Here's the drawing with two shaded views (mm, measured from the low corner). I have some questions. A direction names the side the tool comes from. Coordinates: 2 decimals unless noted, no trailing zeros. Write each loop counter-clockwise with the first axis right and the second up, starting at its lowest first coordinate (ties: lowest second). Pieces come first, ordered by that corner, then holes. Notation, with made-up numbers: M -29.75,56.25 L 4.25,56.25 A27 ccw 4.25,88.25 Z; hole C 8,44.25 d2. An arc over 180 degrees is marked long. Answer as CSV lines item,"result". Start each with the question number.
Item 1: If I drill on line 1 along Y through (x, z) = (17.5, 15); line 2 along Z through (x, y) = (2.5, 28.25); line 3 along X through (y, z) = (6, 11.25), over which ranges is the centre line in solid material (lowest first)? Write a range as [from, to].
Item 2: Suppose I cut it at D-D, the plane z = 1. Write out the boundary of the cut face in (x, y).
Item 3: I'm going to push flat-ended pins straight in: P1, Ø7.5, axis at y = 9, z = 11, coming from the +X side; P2, Ø7.5, axis at y = 6, z = 6, coming from the -X side; P3, Ø4, axis at x = 18.5, z = 10, coming from the -Y side. Where does each tip first touch, or does it pass through?
Item 4: Suppose I cut it at B-B, the plane z = 9.75. Write out the boundary of the cut face in (x, y).
Item 5: Suppose I cut it at C-C, the plane x = 10.25. Write out the boundary of the cut face in (y, z), and give its area (3 significant figures).
Item 6: Suppose I cut it at A-A, the plane y = 6.5. Write out the boundary of the cut face in (x, z).
Item 7: We'd pull the mould along X, two halves only. Please class the marked faces 1, 2, 3 and 4: +X half, -X half, draft (parallel to the pull), parting line (faces both ways), or undercut.
Item 8: On a 3-axis mill with a long thin cutter (end or side, diameter ignored), from which of +Z, -Z, +X, -X, +Y, -Y can I reach the whole of each face in a straight line? I mean the marked faces 5, 6 and 7. Say none if no direction works.
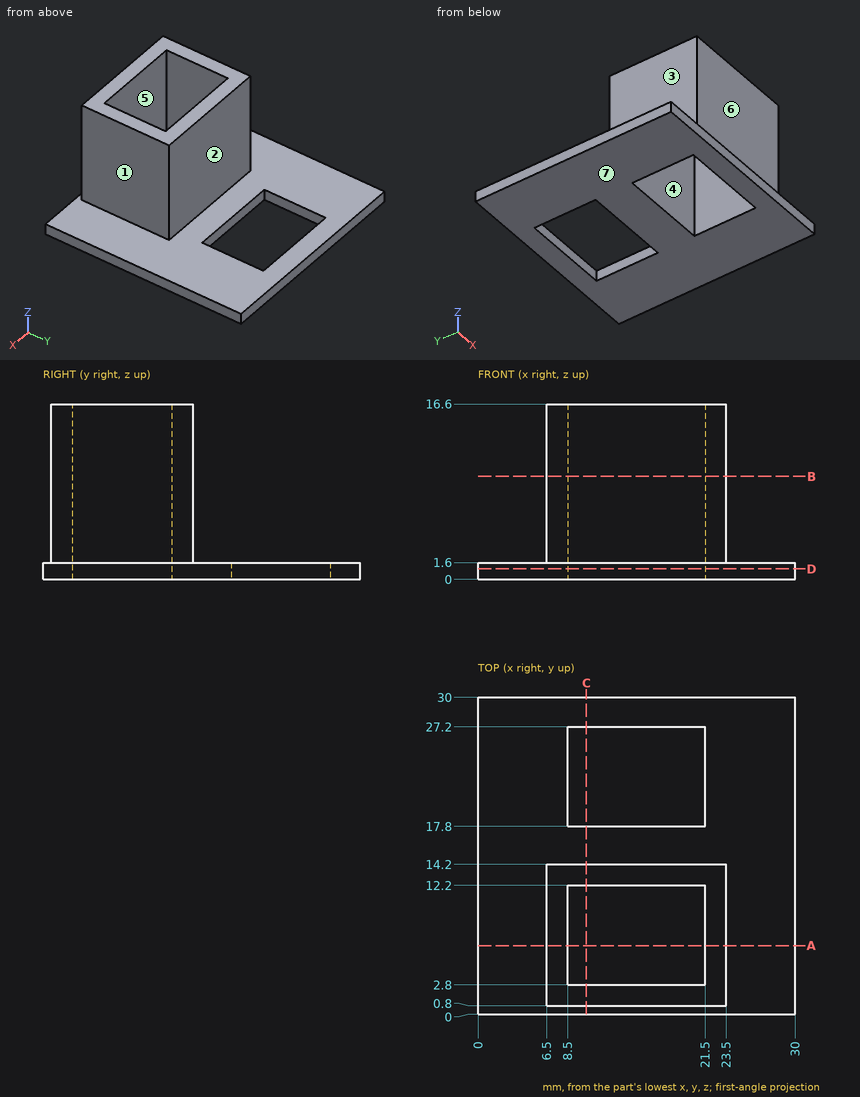
Ans:
1,line 1,"y = [0.8, 2.8], [12.2, 14.2]"
1,line 2,"z = [0, 1.6]"
1,line 3,"x = [6.5, 8.5], [21.5, 23.5]"
2,outline,"M 0,0 L 30,0 L 30,30 L 0,30 Z; hole M 8.5,2.8 L 21.5,2.8 L 21.5,12.2 L 8.5,12.2 Z; hole M 8.5,17.8 L 21.5,17.8 L 21.5,27.2 L 8.5,27.2 Z"
3,P1,"stops at x = 23.5"
3,P2,"stops at x = 6.5"
3,P3,"stops at y = 0.8"
4,outline,"M 6.5,0.8 L 23.5,0.8 L 23.5,14.2 L 6.5,14.2 Z; hole M 8.5,2.8 L 21.5,2.8 L 21.5,12.2 L 8.5,12.2 Z"
5,outline,"M 0,0 L 2.8,0 L 2.8,16.6 L 0.8,16.6 L 0.8,1.6 L 0,1.6 Z; M 12.2,0 L 17.8,0 L 17.8,1.6 L 14.2,1.6 L 14.2,16.6 L 12.2,16.6 Z; M 27.2,0 L 30,0 L 30,1.6 L 27.2,1.6 Z"
5,area,"77.9 mm^2"
6,outline,"M 0,0 L 8.5,0 L 8.5,16.6 L 6.5,16.6 L 6.5,1.6 L 0,1.6 Z; M 21.5,0 L 30,0 L 30,1.6 L 23.5,1.6 L 23.5,16.6 L 21.5,16.6 Z"
7,face 1,"+X half"
7,face 2,"draft"
7,face 3,"-X half"
7,face 4,"undercut"
8,face 5,"+Z, -Z"
8,face 6,"+Z, +X, -X, -Y"
8,face 7,"-Z, +X, -X, +Y, -Y"
